Print and shaded views of the part. All mm, measured from the part's lowest x, y and z. Round coordinates to 2 decimals unless told otherwise and drop trailing zeros. Write each loop counter-clockwise with the first axis right and the second up, starting at its lowest first coordinate (ties: lowest second). Pieces come first, ordered by that corner, then holes. Notation, with made-up numbers: (9, -38.5) -> (36, -38.5) arc R28 cw to (36, -16.5) -> close; hole circle Ø7 at (40.25, 20.25). An arc over 180 degrees is marked (long way). Return JSON: item names as keys, results as strings. Group by question number.
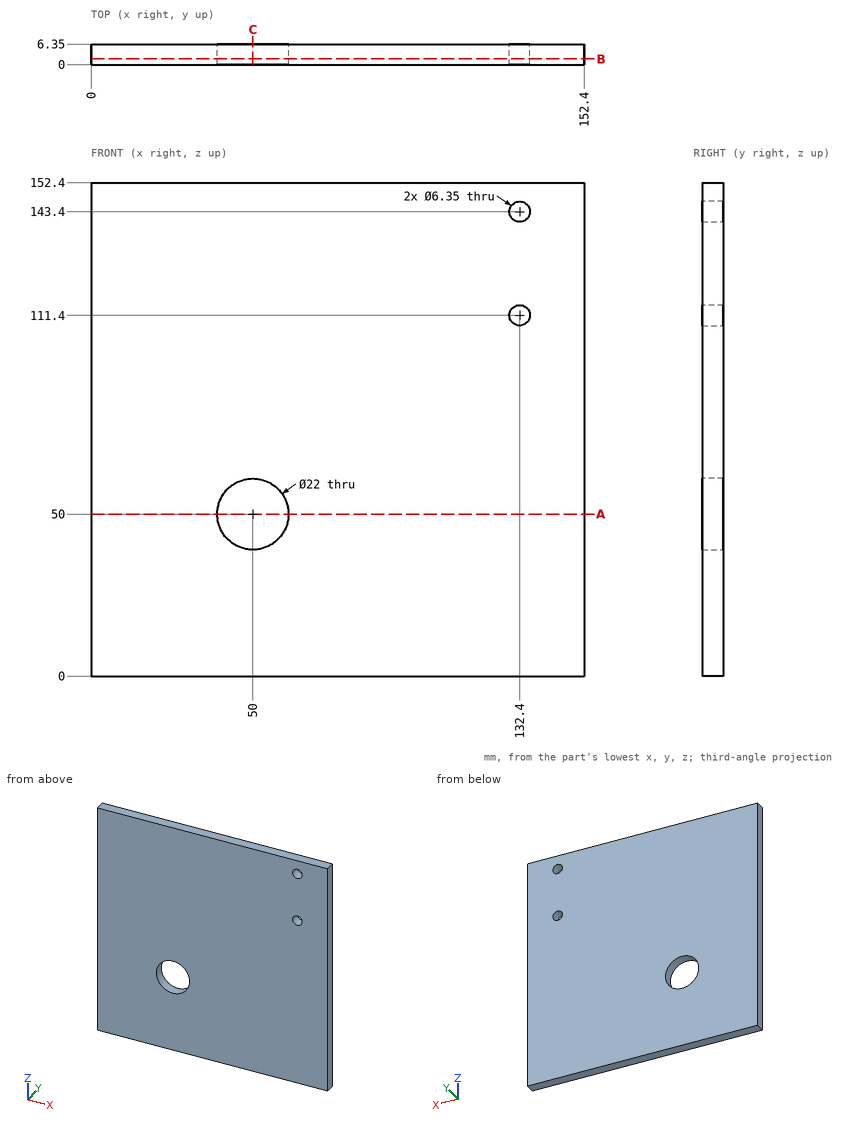
Item 1: Cut at A-A (z = 50). Write the cut outline in (x, y).
Item 2: Cut at B-B (y = 1.75). Write the cut outline in (x, z) (3 decimals), then the cut area to 3 significant figures.
Item 3: Flat gauge pin, fed straight in: P1, Ø5.5, axis at x = 132.4, z = 111.4, coming from the -Y side. Where does the tip first touch, or does it go through?
Item 4: Cut at C-C (x = 50). Write the cut outline in (y, z).
Item 5: Wall check: L1, parallel to Z at x = 132.4, y = 2 (3 decimals); L2, parallel to Z at x = 53.5, y = 5; L3, parallel to Z at x = 48.5, y = 3.5. Give the ranges that are in metal, low to high.
Checks:
{
 "1": {"outline": "(0, 0) -> (39, 0) -> (39, 6.35) -> (0, 6.35) -> close; (61, 0) -> (152.4, 0) -> (152.4, 6.35) -> (61, 6.35) -> close"},
 "2": {"outline": "(0, 0) -> (152.4, 0) -> (152.4, 152.4) -> (0, 152.4) -> close; hole circle Ø22 at (50, 50); hole circle Ø6.35 at (132.4, 111.4); hole circle Ø6.35 at (132.4, 143.4)", "area": "22,800 mm2"},
 "3": {"P1": "passes through"},
 "4": {"outline": "(0, 0) -> (6.35, 0) -> (6.35, 39) -> (0, 39) -> close; (0, 61) -> (6.35, 61) -> (6.35, 152.4) -> (0, 152.4) -> close"},
 "5": {"L1": "z = 0 to 108.225, 114.575 to 140.225, 146.575 to 152.4", "L2": "z = 0 to 39.57, 60.43 to 152.4", "L3": "z = 0 to 39.1, 60.9 to 152.4"}
}
